```python
from build123d import *

# Parameters (mm, degrees)
SKIZZE1_R                             = 44
AUFSATZ_LINEAR_AUSTRAGEN1_DEPTH       = 4
SCHNITT_LINEAR_START                  = -10
SCHNITT_LINEAR_AUSTRAGEN2_DEPTH       = 10
KREISMUSTER1_COUNT                    = 6
SCHNITT_LINEAR_AUSTRAGEN3_DEPTH       = 4
SCHNITT_LINEAR_AUSTRAGEN3_DEPTH_BACK  = 10
VERRUNDUNG1_R                         = 2
SKIZZE7_R                             = 32
SCHNITT_LINEAR_AUSTRAGEN7_DEPTH       = 0.5
SKIZZE8_R                             = 45
SKIZZE8_R_2                           = 43
AUFSATZ_LINEAR_AUSTRAGEN2_DEPTH       = 5
SKIZZE9_R                             = 45
SKIZZE9_R_2                           = 39.5
AUFSATZ_LINEAR_AUSTRAGEN3_DEPTH       = 8
SKIZZE4_R                             = 21.007106764
AUFSATZ_LINEAR_AUSTRAGEN8_DEPTH       = 6
FASE1_SIZE                            = 3.25
SKIZZE10_R                            = 50
SKIZZE10_R_2                          = 42
SCHNITT_LINEAR_AUSTRAGEN9_DEPTH       = 7
SKIZZE11_R                            = 50
SKIZZE11_R_2                          = 40.9
SCHNITT_LINEAR_AUSTRAGEN10_DEPTH      = 2
SCHNITT_LINEAR_AUSTRAGEN11_DEPTH      = 6
SCHNITT_LINEAR_AUSTRAGEN11_DEPTH_BACK = 6
FASE3_SIZE                            = 2
FASE5_SIZE                            = 2


with BuildPart() as part:
    # Skizze1 → Aufsatz-Linear austragen1 (new body)
    with BuildSketch(Plane(origin=(0, 0, 0), x_dir=(1, 0, 0), z_dir=(0, 1, 0))):
        with Locations(Location((0, 0, 0), (0, 0, 270))):
            Circle(SKIZZE1_R)
    extrude(amount=AUFSATZ_LINEAR_AUSTRAGEN1_DEPTH)

    # Skizze2 → Schnitt-Linear austragen2 (cut)
    with BuildSketch(Plane(origin=(0, 4, 0), x_dir=(1, 0, 0), z_dir=(0, 1, 0)).offset(SCHNITT_LINEAR_START)):
        with BuildLine():
            ThreePointArc((-30, 0), (-30.647234858, 7.855929826), (-32.571484726, 15.5))
            Line((-32.571484726, 15.5), (-41.179485184, 15.5))
            ThreePointArc((-41.179485184, 15.5), (-44, 0), (-41.179485184, -15.5))
            Line((-41.179485184, -15.5), (-32.571484726, -15.5))
            ThreePointArc((-32.571484726, -15.5), (-30.647234858, -7.855929826), (-30, 0))
        make_face()
    schnitt_linear_austragen2 = extrude(amount=SCHNITT_LINEAR_AUSTRAGEN2_DEPTH, mode=Mode.SUBTRACT)

    # Kreismuster1: Schnitt-Linear austragen2 ×6 about axis
    kreismuster1_axis = Axis((0, 0, 0), (0, 1, 0))
    for i in range(1, KREISMUSTER1_COUNT):
        add(schnitt_linear_austragen2.rotate(kreismuster1_axis, i * 360 / KREISMUSTER1_COUNT), mode=Mode.SUBTRACT)

    # Skizze3 → Schnitt-Linear austragen3 (cut, two sides: drawn at the far end of the back side and taken through both)
    with BuildSketch(Plane.XZ.offset(-SCHNITT_LINEAR_AUSTRAGEN3_DEPTH_BACK)):
        Polygon((15, 8.660254038), (0, 17.320508076), (-15, 8.660254038), (-15, -8.660254038), (0, -17.320508076), (15, -8.660254038), align=None)
    extrude(amount=SCHNITT_LINEAR_AUSTRAGEN3_DEPTH + SCHNITT_LINEAR_AUSTRAGEN3_DEPTH_BACK, mode=Mode.SUBTRACT)

    # Verrundung1
    verrundung1_edges = [part.edges().sort_by_distance(p)[0] for p in [
        (-32.571484726, 2, 15.5),
        (-32.571484726, 2, -15.5),
        (-29.709136122, 2, -20.457733212),
        (-2.862348604, 2, -35.957733212),
        (2.862348604, 2, -35.957733212),
        (29.709136122, 2, -20.457733212),
        (32.571484726, 2, -15.5),
        (32.571484726, 2, 15.5),
        (29.709136122, 2, 20.457733212),
        (2.862348604, 2, 35.957733212),
        (-2.862348604, 2, 35.957733212),
        (-29.709136122, 2, 20.457733212),
    ]]
    fillet(verrundung1_edges, radius=VERRUNDUNG1_R)

    # Skizze7 → Schnitt-Linear austragen7 (cut)
    with BuildSketch(Plane.XZ):
        Circle(SKIZZE7_R)
    extrude(amount=-SCHNITT_LINEAR_AUSTRAGEN7_DEPTH, mode=Mode.SUBTRACT)

    # Skizze8 → Aufsatz-Linear austragen2 (add)
    with BuildSketch(Plane(origin=(0, 4, 0), x_dir=(1, 0, 0), z_dir=(0, 1, 0))):
        with Locations(Location((0, 0, 0), (0, 0, 270))):
            Circle(SKIZZE8_R)
        with Locations(Location((0, 0, 0), (0, 0, 270))):
            Circle(SKIZZE8_R_2, mode=Mode.SUBTRACT)
    extrude(amount=-AUFSATZ_LINEAR_AUSTRAGEN2_DEPTH)



with BuildPart() as body_2:
    # Skizze9 → Aufsatz-Linear austragen3 (new body)
    with BuildSketch(Plane.XZ.offset(1)):
        with Locations(Location((0, 0, 0), (0, 0, 90))):
            Circle(SKIZZE9_R)
        with Locations(Location((0, 0, 0), (0, 0, 270))):
            Circle(SKIZZE9_R_2, mode=Mode.SUBTRACT)
    extrude(amount=AUFSATZ_LINEAR_AUSTRAGEN3_DEPTH)


with BuildPart() as part_1:
    add(part.part)

    add(body_2.part)  # Aufsatz-Linear austragen8 merges body 2
    # Skizze4 → Aufsatz-Linear austragen8 (add)
    with BuildSketch(Plane(origin=(0, 4, 0), x_dir=(1, 0, 0), z_dir=(0, 1, 0))):
        with Locations(Location((0, 0, 0), (0, 0, 270))):
            Circle(SKIZZE4_R)
    extrude(amount=-AUFSATZ_LINEAR_AUSTRAGEN8_DEPTH)

    # Fase1
    fase1_edges = [part_1.edges().sort_by_distance(p)[0] for p in [
        (0, -1, 39.5),
    ]]
    chamfer(fase1_edges, length=FASE1_SIZE)

    # Skizze10 → Schnitt-Linear austragen9 (cut)
    with BuildSketch(Plane.XZ.offset(9)):
        Circle(SKIZZE10_R)
        with Locations(Location((0, 0, 0), (0, 0, 270))):
            Circle(SKIZZE10_R_2, mode=Mode.SUBTRACT)
    extrude(amount=-SCHNITT_LINEAR_AUSTRAGEN9_DEPTH, mode=Mode.SUBTRACT)

    # Skizze11 → Schnitt-Linear austragen10 (cut)
    with BuildSketch(Plane.XZ.offset(9)):
        with Locations((-1.948563864, 1.772578218)):
            Circle(SKIZZE11_R)
        with Locations(Location((0, 0, 0), (0, 0, 270))):
            Circle(SKIZZE11_R_2, mode=Mode.SUBTRACT)
    extrude(amount=-SCHNITT_LINEAR_AUSTRAGEN10_DEPTH, mode=Mode.SUBTRACT)

    # Skizze3_3 → Schnitt-Linear austragen11 (cut, two sides: drawn at the far end of the back side and taken through both)
    with BuildSketch(Plane.XZ.offset(-SCHNITT_LINEAR_AUSTRAGEN11_DEPTH_BACK)):
        Polygon((15, 8.660254038), (0, 17.320508076), (-15, 8.660254038), (-15, -8.660254038), (0, -17.320508076), (15, -8.660254038), align=None)
    extrude(amount=SCHNITT_LINEAR_AUSTRAGEN11_DEPTH + SCHNITT_LINEAR_AUSTRAGEN11_DEPTH_BACK, mode=Mode.SUBTRACT)

    # Fase3
    fase3_edges = [part_1.edges().sort_by_distance(p)[0] for p in [
        (0, -2, -21.007106764),
    ]]
    chamfer(fase3_edges, length=FASE3_SIZE)

    # Fase5
    fase5_edges = [part_1.edges().sort_by_distance(p)[0] for p in [
        (15, 4, 0),
        (7.5, 4, 12.990381057),
        (-7.5, 4, 12.990381057),
        (-15, 4, 0),
        (-7.5, 4, -12.990381057),
        (7.5, 4, -12.990381057),
    ]]
    chamfer(fase5_edges, length=FASE5_SIZE)


solid = part_1.part
```
Build history of the part. All positions in model axes, mm. A direction names the side the tool comes from. Coordinates: 2 decimals unless noted, no trailing zeros.
1. Band-saw the part on A-A, the plane x = 5. Give the number of separate pieces and of enclosed holes in the cut face, and give its area (3 significant figures).
Answer block:
separate pieces: 4
enclosed holes: 0
area: 234 mm2
2. Pull direction X, two halves, no side cores. Call faces 1 (the cylindrical face through (17.235, 1.042, 41.569)), 2 (the flat face through (37, 2, 15.5)), 3 (the flat face through (-14, -2, -40)): released by +X, released by -X, zero draft, split by the parting line, or undercut.
Answer block:
face 1: split by the parting line
face 2: undercut
face 3: zero draft
3. 3-axis set-ups, long thin cutter, end or side, ignore diameter. For faces 4 (the flat face through (-31.936, 1.972, 24.314)), 5 (the flat face through (0, 0.5, 22)), 6 (the cylindrical face through (-29.52, 2.03, -20.89)): which of +Z, -Z, +X, -X, +Y, -Y reach the whole face in a straight line?
Answer block:
face 4: +Y
face 5: -Y
face 6: +Y, -Y
4. Drill centre lines: probe 1 along X at (y, z) = (0.25, 0); probe 2 along X at (y, z) = (-7.25, -0.5); probe 3 along X at (y, z) = (-0.75, 14). Where is each one in solid material? Low to high.
Answer block:
probe 1: x = -45 to -43, -21.01 to -15, 15 to 21.01, 43 to 45
probe 2: x = -40.9 to -39.5, 39.5 to 40.9
probe 3: x = -42.77 to -40.66, -14.64 to -5.75, 5.75 to 14.64, 40.66 to 42.77
5. Drop flat-ended pins along their axis: pin 1 (4 mm diameter, centred on x = 34.5, y = 1.5, fed in from +Z); pin 2 (2 mm diameter, centred on x = -16, y = -0.5, fed in from +Z); pin 3 (1.2 mm diameter, centred on y = 0, z = -1, fed in from +X). Give the stop position or say it passes through.
Answer block:
pin 1: stops at z = 31.12
pin 2: stops at z = 42.43
pin 3: stops at x = 45
